For this review, take the finished solid that the model builds, in its own axes (mm). Face numbers are marked on the shaded views. A direction names the side the tool comes from. Coordinates: 2 decimals unless noted, no trailing zeros. Order: outer loops, then holes, each group sorted by start corner. A loop starts at its lowest first (then second) coordinate and runs counter-clockwise, first axis right, second up. Notation, with made-up numbers: (71.5, 56.25) -> (117.5, 56.25) arc R32 cw to (117.5, 88.25) -> close; hole circle Ø9 at (55.5, 4). An arc over 180 degrees is marked (long way). Return JSON: item names as keys, results as strings. Group by question number.
Item 1: Insertion check: pin 1 (8 mm diameter, centred on x = -10.5, y = 12.5, fed in from +Z); pin 2 (1.5 mm diameter, centred on x = -3.5, y = 5.5, fed in from -Z); pin 3 (0.6 mm diameter, centred on y = 7, z = 14.5, fed in from -X). Each pin has a flat end and moves straight along its axis. Give the tip position at first contact, or say it passes through.
Item 2: Take a section at C-C (z = 60). Write out the cut boundary in (x, y), then the cut area to 3 significant figures.
Item 3: For line 1 along Z through (x, y) = (-6.5, 7.5); line 2 along Z through (x, y) = (-9, 6.5); line 3 along Y through (x, z) = (-8, 17), list the stretches that pass through material, from the lowest coordinate up.
Item 4: Take a section at B-B (y = 11.25). Write out the cut boundary in (x, z).
Item 5: Take a section at A-A (x = -11.5). Write out the cut boundary in (y, z), then the cut area to 3 significant figures.
Item 6: Machinability: for the marked faces 1, 2 and 3, which of the approach directions +Z, -Z, +X, -X, +Y, -Y give a long, thin tool a straight path to every point of the face, cutting with its end or side? Answer none if there is none.
Item 7: Take a section at D-D (x = -3.25). Write out the cut boundary in (y, z).
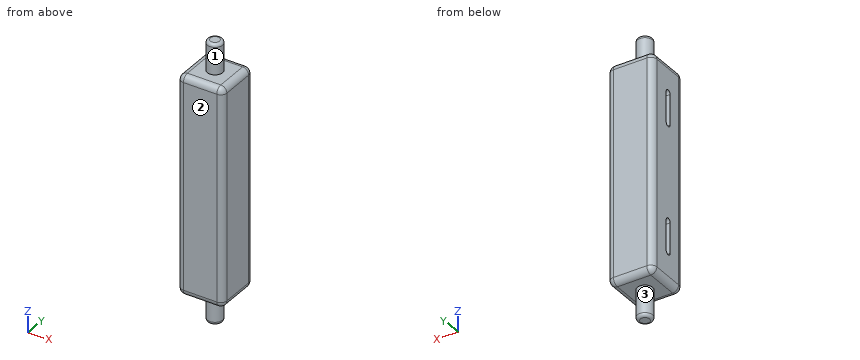
```python
from build123d import *

# Parameters (mm, degrees)
SKETCH1_W           = 15
SKETCH1_H           = 15
BOSS_EXTRUDE1_DEPTH = 72
SKETCH2_R           = 2.5
BOSS_EXTRUDE2_DEPTH = 10
BOSS_EXTRUDE3_START = 10
SKETCH3_R           = 2.5
BOSS_EXTRUDE3_DEPTH = 10
CUT_EXTRUDE1_DEPTH  = 10
FILLET1_R           = 2
FILLET2_R           = 2
FILLET3_R           = 2
FILLET4_R           = 2
FILLET5_R           = 2
FILLET6_R           = 2
FILLET7_R           = 1
FILLET8_R           = 1


with BuildPart() as part:
    # Sketch1 → Boss-Extrude1 (new body)
    with BuildSketch(Plane.XY):
        with Locations((-7.5, 7.5)):
            Rectangle(SKETCH1_W, SKETCH1_H)
    extrude(amount=BOSS_EXTRUDE1_DEPTH)

    # Sketch2 → Boss-Extrude2 (add)
    with BuildSketch(Plane(origin=(0, 0, 0), x_dir=(-1, 0, 0), z_dir=(0, 0, -1))):
        with Locations((7.5, 7.5)):
            Circle(SKETCH2_R)
    extrude(amount=BOSS_EXTRUDE2_DEPTH)

    # Sketch3 → Boss-Extrude3 (add)
    with BuildSketch(Plane.XY.offset(72).offset(BOSS_EXTRUDE3_START)):
        with Locations(Location((-7.5, 7.5, 0), (0, 0, 180))):
            Circle(SKETCH3_R)
    extrude(amount=-BOSS_EXTRUDE3_DEPTH)

    # Sketch5 → Cut-Extrude1 (cut)
    with BuildSketch(Plane.ZY.offset(15)):
        with BuildLine():
            Line((20, 6.306366703), (10, 6.306366703))
            ThreePointArc((10, 6.306366703), (9, 7.306366703), (10, 8.306366703))
            Line((10, 8.306366703), (20, 8.306366703))
            ThreePointArc((20, 8.306366703), (21, 7.306366703), (20, 6.306366703))
        make_face()
        with BuildLine():
            Line((52, 8.306366703), (62, 8.306366703))
            ThreePointArc((62, 8.306366703), (63, 7.306366703), (62, 6.306366703))
            Line((62, 6.306366703), (52, 6.306366703))
            ThreePointArc((52, 6.306366703), (51, 7.306366703), (52, 8.306366703))
        make_face()
    extrude(amount=-CUT_EXTRUDE1_DEPTH, mode=Mode.SUBTRACT)

    # Fillet1
    fillet1_edges = [part.edges().sort_by_distance(p)[0] for p in [
        (-15, 15, 36),
    ]]
    fillet(fillet1_edges, radius=FILLET1_R)

    # Fillet2
    fillet2_edges = [part.edges().sort_by_distance(p)[0] for p in [
        (0, 15, 36),
    ]]
    fillet(fillet2_edges, radius=FILLET2_R)

    # Fillet3
    fillet3_edges = [part.edges().sort_by_distance(p)[0] for p in [
        (0, 0, 36),
    ]]
    fillet(fillet3_edges, radius=FILLET3_R)

    # Fillet4
    fillet4_edges = [part.edges().sort_by_distance(p)[0] for p in [
        (-15, 0, 36),
    ]]
    fillet(fillet4_edges, radius=FILLET4_R)

    # Fillet5
    fillet5_edges = [part.edges().sort_by_distance(p)[0] for p in [
        (-15, 7.5, 0),
        (-14.414213562, 14.414213562, 0),
        (-7.5, 15, 0),
        (-0.585786438, 14.414213562, 0),
        (0, 7.5, 0),
        (-0.585786438, 0.585786438, 0),
        (-7.5, 0, 0),
        (-14.414213562, 0.585786438, 0),
    ]]
    fillet(fillet5_edges, radius=FILLET5_R)

    # Fillet6
    fillet6_edges = [part.edges().sort_by_distance(p)[0] for p in [
        (-15, 7.5, 72),
        (-14.414213562, 14.414213562, 72),
        (-7.5, 15, 72),
        (-0.585786438, 14.414213562, 72),
        (0, 7.5, 72),
        (-0.585786438, 0.585786438, 72),
        (-7.5, 0, 72),
        (-14.414213562, 0.585786438, 72),
    ]]
    fillet(fillet6_edges, radius=FILLET6_R)

    # Fillet7
    fillet7_edges = [part.edges().sort_by_distance(p)[0] for p in [
        (-5, 7.5, 82),
    ]]
    fillet(fillet7_edges, radius=FILLET7_R)

    # Fillet8
    fillet8_edges = [part.edges().sort_by_distance(p)[0] for p in [
        (-5, 7.5, -10),
    ]]
    fillet(fillet8_edges, radius=FILLET8_R)


solid = part.part
```
Findings below:
{
 "1": {"pin 1": "stops at z = 81.94", "pin 2": "stops at z = 0", "pin 3": "stops at x = -5"},
 "2": {"outline": "(-15, 2) arc R2 ccw to (-13, 0) -> (-2, 0) arc R2 ccw to (0, 2) -> (0, 13) arc R2 ccw to (-2, 15) -> (-13, 15) arc R2 ccw to (-15, 13) -> (-15, 8.31) -> (-5, 8.31) -> (-5, 6.31) -> (-15, 6.31) -> close", "area": "202 mm2"},
 "3": {"line 1": "z = -10 to 9.02, 20.98 to 51.02, 62.98 to 82", "line 2": "z = -9.95 to 9.41, 20.59 to 51.41, 62.59 to 81.95", "line 3": "y = 0 to 6.31, 8.31 to 15"},
 "4": {"outline": "(-15, 2) arc R2 ccw to (-13, 0) -> (-2, 0) arc R2 ccw to (0, 2) -> (0, 70) arc R2 ccw to (-2, 72) -> (-13, 72) arc R2 ccw to (-15, 70) -> close"},
 "5": {"outline": "(0, 2) arc R2 ccw to (2, 0) -> (13, 0) arc R2 ccw to (15, 2) -> (15, 70) arc R2 ccw to (13, 72) -> (2, 72) arc R2 ccw to (0, 70) -> close; hole (6.31, 10) arc R1 ccw to (8.31, 10) -> (8.31, 20) arc R1 ccw to (6.31, 20) -> close; hole (6.31, 52) arc R1 ccw to (8.31, 52) -> (8.31, 62) arc R1 ccw to (6.31, 62) -> close", "area": "1,030 mm2"},
 "6": {"face 1": "+Z", "face 2": "+Z, -Z, +X, -X, -Y", "face 3": "-Z"},
 "7": {"outline": "(0, 2) arc R2 ccw to (2, 0) -> (13, 0) arc R2 ccw to (15, 2) -> (15, 70) arc R2 ccw to (13, 72) -> (2, 72) arc R2 ccw to (0, 70) -> close"}
}
